Verification items for the finished model (mm, model axes). Coordinates: 2 decimals unless noted, no trailing zeros. Write each loop counter-clockwise with the first axis right and the second up, starting at its lowest first coordinate (ties: lowest second). Pieces come first, ordered by that corner, then holes. Notation, with made-up numbers: M -26,63 L 31,63 A9 ccw 31,79 Z; hole C 45.5,28.25 d4. An arc over 180 degrees is marked long. One line per item, written item: value.
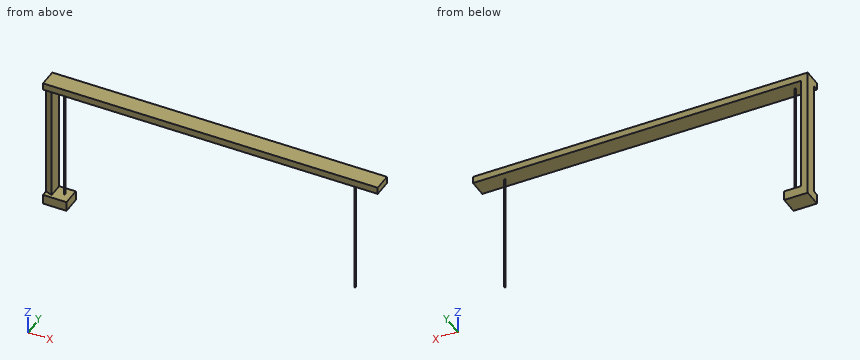
```python
from build123d import *

# Parameters (mm, degrees)
SKETCH1_W           = 25
SKETCH1_H           = 13
BOSS_EXTRUDE1_DEPTH = 5
SKETCH2_R           = 0.4
BOSS_EXTRUDE2_DEPTH = 87
SKETCH3_W           = 5
SKETCH3_H           = 13
BOSS_EXTRUDE3_DEPTH = 210
SKETCH4_R           = 0.4
BOSS_EXTRUDE4_DEPTH = 87
SKETCH5_W           = 5
SKETCH5_H           = 13
BOSS_EXTRUDE5_DEPTH = 7
SKETCH6_W           = 5
SKETCH6_H           = 13
BOSS_EXTRUDE6_DEPTH = 92
BOSS_EXTRUDE7_START = -13
SKETCH8_W           = 12
SKETCH8_H           = 7
BOSS_EXTRUDE7_DEPTH = 13
CUT_EXTRUDE4_DEPTH  = 85


with BuildPart() as part:
    # Sketch1 → Boss-Extrude1 (new body)
    with BuildSketch(Plane.XY):
        with Locations((12.5, 6.5)):
            Rectangle(SKETCH1_W, SKETCH1_H)
    extrude(amount=BOSS_EXTRUDE1_DEPTH)

    # Sketch2 → Boss-Extrude2 (add)
    with BuildSketch(Plane(origin=(0, 0, 0), x_dir=(-1, 0, 0), z_dir=(0, 0, -1))):
        with Locations((-5, 7.1)):
            Circle(SKETCH2_R)
    extrude(amount=BOSS_EXTRUDE2_DEPTH)

    # Sketch3 → Boss-Extrude3 (add)
    with BuildSketch(Plane.ZY):
        with Locations((2.5, 6.5)):
            Rectangle(SKETCH3_W, SKETCH3_H)
    extrude(amount=BOSS_EXTRUDE3_DEPTH)

    # Sketch4 → Boss-Extrude4 (add)
    with BuildSketch(Plane(origin=(0, 0, 0), x_dir=(-1, 0, 0), z_dir=(0, 0, -1))):
        with Locations((205, 7.1)):
            Circle(SKETCH4_R)
    extrude(amount=BOSS_EXTRUDE4_DEPTH)

    # Sketch5 → Boss-Extrude5 (add)
    with BuildSketch(Plane.ZY.offset(210)):
        with Locations((2.5, 6.5)):
            Rectangle(SKETCH5_W, SKETCH5_H)
    extrude(amount=BOSS_EXTRUDE5_DEPTH)

    # Sketch6 → Boss-Extrude6 (add)
    with BuildSketch(Plane(origin=(0, 0, 0), x_dir=(-1, 0, 0), z_dir=(0, 0, -1))):
        with Locations((214.5, 6.5)):
            Rectangle(SKETCH6_W, SKETCH6_H)
    extrude(amount=BOSS_EXTRUDE6_DEPTH)

    # Sketch8 → Boss-Extrude7 (add)
    with BuildSketch(Plane.XZ.offset(BOSS_EXTRUDE7_START)):
        with Locations((-206, -88.5)):
            Rectangle(SKETCH8_W, SKETCH8_H)
    extrude(amount=BOSS_EXTRUDE7_DEPTH)

    # Sketch12 → Cut-Extrude4 (cut)
    with BuildSketch(Plane(origin=(0, 0, 0), x_dir=(-1, 0, 0), z_dir=(0, 0, -1))):
        Polygon((204.365486279, 0), (217, 4.113001179), (217, 0), align=None)
    extrude(amount=CUT_EXTRUDE4_DEPTH, mode=Mode.SUBTRACT)


solid = part.part
```
Item 1: Cross-section at B-B, the plane x = -67. Enter the section's corners in (y, z), and give its area (3 significant figures).
The answers:
outline: M 0,0 L 13,0 L 13,5 L 0,5 Z
area: 65.0 mm²
Item 2: Go/stop test with flat-tipped pins: P1, Ø8, axis at x = -4, z = -6.5, coming from the +Y side; P2, Ø5.5, axis at y = 8.5, z = -35.5, coming from the +X side; P3, Ø0.9, axis at x = 5, y = 7, coming from the -Z side; P4, Ø5, axis at x = -178.5, y = 6.5, coming from the -Z side. Record where each tip stops, or that it passes through.
The answers:
P1: passes through
P2: stops at x = 5.4
P3: stops at z = -87
P4: stops at z = 0
Item 3: Cross-section at A-A, the plane z = -74. Enter the section's corners in (x, y), and give its area (3 significant figures).
The answers:
outline: M -217,4.11 L -212,2.49 L -212,13 L -217,13 Z; C -205,7.1 d0.8; C 5,7.1 d0.8
area: 49.5 mm²
Item 4: Scan lines: line 1 (X direction, y = 7.25, z = -9); line 2 (Z direction, x = -12, y = 9.5); line 3 (Z direction, x = -203.5, y = 9). Record each from-to range of solid material in increasing order.
The answers:
line 1: x = -217 to -212, -205.37 to -204.63, 4.63 to 5.37
line 2: z = 0 to 5
line 3: z = -92 to -85, 0 to 5
